```python
from build123d import *

# Parameters (mm, degrees)
SALIENTE_EXTRUIR1_DEPTH    = 100
VACIADO2_T                 = -2
CROQUIS2_R                 = 1.5
CORTAR_EXTRUIR1_DEPTH      = 101
CORTAR_EXTRUIR1_DEPTH_BACK = 1
CROQUIS8_R                 = 28
CROQUIS8_R_2               = 1.5
CORTAR_EXTRUIR6_DEPTH      = 130.862159322
CORTAR_EXTRUIR7_DEPTH      = 113.5
CORTAR_EXTRUIR8_DEPTH      = 86
CORTAR_EXTRUIR8_DEPTH_BACK = 86
CROQUIS11_R                = 29
CROQUIS11_R_2              = 2
CORTAR_EXTRUIR9_DEPTH      = 113.5


with BuildPart() as part:
    # Croquis1 → Saliente-Extruir1 (new body)
    with BuildSketch(Plane(origin=(0, 0, 0), x_dir=(1, 0, 0), z_dir=(0, 1, 0))):
        with BuildLine():
            Line((-82.320508076, 47.858983849), (-50.773502692, 102.5))
            ThreePointArc((-50.773502692, 102.5), (-43.452994616, 109.820508076), (-33.452994616, 112.5))
            Line((-33.452994616, 112.5), (33.452994616, 112.5))
            ThreePointArc((33.452994616, 112.5), (43.452994616, 109.820508076), (50.773502692, 102.5))
            Line((50.773502692, 102.5), (82.320508076, 47.858983849))
            ThreePointArc((82.320508076, 47.858983849), (84.318516526, 43.035364751), (85, 37.858983849))
            Line((85, 37.858983849), (85, -37.858983849))
            ThreePointArc((85, -37.858983849), (84.318516526, -43.035364751), (82.320508076, -47.858983849))
            Line((82.320508076, -47.858983849), (50.773502692, -102.5))
            ThreePointArc((50.773502692, -102.5), (43.452994616, -109.820508076), (33.452994616, -112.5))
            Line((33.452994616, -112.5), (-33.452994616, -112.5))
            ThreePointArc((-33.452994616, -112.5), (-43.452994616, -109.820508076), (-50.773502692, -102.5))
            Line((-50.773502692, -102.5), (-82.320508076, -47.858983849))
            ThreePointArc((-82.320508076, -47.858983849), (-84.318516526, -43.035364751), (-85, -37.858983849))
            Line((-85, -37.858983849), (-85, 37.858983849))
            ThreePointArc((-85, 37.858983849), (-84.318516526, 43.035364751), (-82.320508076, 47.858983849))
        make_face()
    extrude(amount=SALIENTE_EXTRUIR1_DEPTH)

    # Vaciado2
    vaciado2_openings = [part.faces().sort_by_distance(p)[0] for p in [
        (0, 100, 0),
    ]]
    offset(amount=VACIADO2_T, openings=vaciado2_openings, kind=Kind.INTERSECTION)

    # Croquis2 → Cortar-Extruir1 (cut, two sides)
    with BuildSketch(Plane(origin=(0, 0, 0), x_dir=(1, 0, 0), z_dir=(0, 1, 0))) as cortar_extruir1_sk:
        with Locations((-45.75, 76.25)):
            Circle(CROQUIS2_R)
        with Locations((-45.75, 58.75)):
            Circle(CROQUIS2_R)
        with Locations((45.75, 58.75)):
            Circle(CROQUIS2_R)
        with Locations((-45.75, -58.75)):
            Circle(CROQUIS2_R)
        with Locations((45.75, -58.75)):
            Circle(CROQUIS2_R)
        with Locations((45.75, -76.25)):
            Circle(CROQUIS2_R)
    extrude(amount=CORTAR_EXTRUIR1_DEPTH, mode=Mode.SUBTRACT)
    extrude(cortar_extruir1_sk.sketch, amount=-CORTAR_EXTRUIR1_DEPTH_BACK, mode=Mode.SUBTRACT)

    # Croquis8 → Cortar-Extruir6 (cut, through all)
    with BuildSketch(Plane(origin=(0, 0, 0), x_dir=(-0.5, 0, -0.866025404), z_dir=(0.866025404, 0, -0.5))):
        with Locations((31.833847158, 40)):
            Circle(CROQUIS8_R)
        with Locations((6.833847158, 65)):
            Circle(CROQUIS8_R_2)
        with Locations((56.833847158, 65)):
            Circle(CROQUIS8_R_2)
        with Locations((6.833847158, 15)):
            Circle(CROQUIS8_R_2)
        with Locations((56.833847158, 15)):
            Circle(CROQUIS8_R_2)
    cortar_extruir6 = extrude(amount=CORTAR_EXTRUIR6_DEPTH, mode=Mode.SUBTRACT)

    # Simetría1: Cortar-Extruir6 across plane
    add(cortar_extruir6.mirror(Plane(origin=(0, 0, 0), x_dir=(0, 0, 1), z_dir=(1, 0, 0))), mode=Mode.SUBTRACT)

    # Croquis9 → Cortar-Extruir7 (cut, through all)
    with BuildSketch(Plane.XY):
        with BuildLine():
            Line((17.5, 55), (-17.5, 55))
            ThreePointArc((-17.5, 55), (-21.035533906, 53.535533906), (-22.5, 50))
            Line((-22.5, 50), (-22.5, 35))
            ThreePointArc((-22.5, 35), (-21.035533906, 31.464466094), (-17.5, 30))
            Line((-17.5, 30), (17.5, 30))
            ThreePointArc((17.5, 30), (21.035533906, 31.464466094), (22.5, 35))
            Line((22.5, 35), (22.5, 50))
            ThreePointArc((22.5, 50), (21.035533906, 53.535533906), (17.5, 55))
        make_face()
    extrude(amount=-CORTAR_EXTRUIR7_DEPTH, mode=Mode.SUBTRACT)

    # Croquis10 → Cortar-Extruir8 (cut, two sides)
    with BuildSketch(Plane(origin=(0, 0, 0), x_dir=(0, 0, -1), z_dir=(1, 0, 0))) as cortar_extruir8_sk:
        Polygon((0, 100), (-148.82762011, 60.12175938), (-148.82762011, 114.287226581), (0, 114.287226581), align=None)
    extrude(amount=CORTAR_EXTRUIR8_DEPTH, mode=Mode.SUBTRACT)
    extrude(cortar_extruir8_sk.sketch, amount=-CORTAR_EXTRUIR8_DEPTH_BACK, mode=Mode.SUBTRACT)

    # Croquis11 → Cortar-Extruir9 (cut, through all)
    with BuildSketch(Plane.XY):
        with Locations((0, 35)):
            Circle(CROQUIS11_R)
        with Locations((25, 10)):
            Circle(CROQUIS11_R_2)
        with Locations((-25, 10)):
            Circle(CROQUIS11_R_2)
        with Locations((-25, 60)):
            Circle(CROQUIS11_R_2)
        with Locations((25, 60)):
            Circle(CROQUIS11_R_2)
    extrude(amount=CORTAR_EXTRUIR9_DEPTH, mode=Mode.SUBTRACT)


solid = part.part
```
Design review of the part built by this model. Coordinates are the model's own, in mm. A direction names the side the tool comes from. Give positions to 0.01 mm unless a question says otherwise; leave off trailing zeros. Loops run counter-clockwise (first coordinate to the right, second up) from the corner with the lowest first, then second, coordinate; pieces in that order, holes last. Notation, with made-up numbers: (77, 65.5) -> (136, 65.5) arc R23 cw to (136, 103.5) -> close; hole circle Ø10 at (85, -7). An arc over 180 degrees is marked (long way). One line per item, written item: value.
Q1. Machinability: for faces 1 (the flat face through (0, 60, -112.5)), 2 (the cylindrical face through (42.57, 36.91, 108.02)), 3 (the flat face through (-29.3, 34.4, 112.5)), 4 (the cylindrical face through (21, 31.43, -111.49)), 5 (the cylindrical face through (15.59, 59.453, 111.486)), which of the approach directions +Z, -Z, +X, -X, +Y, -Y give a long, thin tool a straight path to every point of the face, cutting with its end or side? Answer none if there is none.
Numbers:
face 1: -Z, +X, -X, +Y, -Y
face 2: +Y
face 3: +Z, +X, -X, +Y, -Y
face 4: +Z, -Z
face 5: +Z
Q2. Draft analysis for pull direction Y (two halves, no side actions). For faces 6 (the flat face through (1, 2, -2)), 7 (the cylindrical face through (-21, 53.57, -111.49)), 8 (the flat face through (-66.768, 71.522, -74.797)), state which applies: pulls with the +Y half, pulls with the -Y half, needs draft (parallel to the pull), parting line crosses it, or undercut.
Numbers:
face 6: pulls with the +Y half
face 7: undercut
face 8: needs draft
Q3. We need section A-A on z = -4. Give the boundary of the cut face in (x, y), and give its area (3 significant figures).
Numbers:
outline: (-85, 0) -> (85, 0) -> (85, 100) -> (83, 100) -> (83, 2) -> (-83, 2) -> (-83, 100) -> (-85, 100) -> close
area: 732 mm^2
Q4. We need section B-B on y = 75.5. Give the boundary of the cut face in (x, z).
Numbers:
outline: (-85, -37.86) arc R20 ccw to (-82.32, -47.86) -> (-50.77, -102.5) arc R20 ccw to (-33.45, -112.5) -> (33.45, -112.5) arc R20 ccw to (50.77, -102.5) -> (82.32, -47.86) arc R20 ccw to (85, -37.86) -> (85, 37.86) arc R20 ccw to (82.32, 47.86) -> (57.16, 91.44) -> (54.85, 91.44) -> (80.59, 46.86) arc R18 cw to (83, 37.86) -> (83, -37.86) arc R18 cw to (80.59, -46.86) -> (49.04, -101.5) arc R18 cw to (33.45, -110.5) -> (-33.45, -110.5) arc R18 cw to (-49.04, -101.5) -> (-80.59, -46.86) arc R18 cw to (-83, -37.86) -> (-83, 37.86) arc R18 cw to (-80.59, 46.86) -> (-54.85, 91.44) -> (-57.16, 91.44) -> (-82.32, 47.86) arc R20 ccw to (-85, 37.86) -> close
Q5. We need section C-C on z = 65.5. Give the boundary of the cut face in (x, y).
Numbers:
outline: (-72.14, 0) -> (72.14, 0) -> (72.14, 82.45) -> (69.83, 82.45) -> (69.83, 2) -> (-69.83, 2) -> (-69.83, 82.45) -> (-72.14, 82.45) -> close
Q6. For pin 1 Ø0.6 at (x, z) = (1, -112) entering from -Y; pin 2 Ø1.5 at (x, y) = (-66.5, 60) entering from +Z; pin 3 Ø10 at (y, z) = (53.5, 87.5) entering from -X; pin 4 Ø3.5 at (x, y) = (25, 10) entering from +Z, all flat-tipped, find the tip position at first contact; note any pin that passes through.
Numbers:
pin 1: stops at y = 0
pin 2: stops at z = 76.56
pin 3: stops at x = -62.32
pin 4: stops at z = -110.5
Q7. For L1, parallel to X at y = 61, z = 11; L2, parallel to X at y = 60, z = 111; L3, parallel to Z at x = 28, y = 57, list the stretches that pass through material, from the lowest coordinate up.
Numbers:
L1: x = -85 to -83, 83 to 85
L2: x = -41.05 to -27, -23 to -14.7, 14.7 to 23, 27 to 41.05
L3: z = -112.5 to -110.5, 110.5 to 112.5
